Geometry check sheet. Reference: the model listing, model coordinates, mm. Face numbers are marked on the shaded views. A direction names the side the tool comes from. Give positions to 0.01 mm unless a question says otherwise; leave off trailing zeros. Write each loop counter-clockwise with the first axis right and the second up, starting at its lowest first coordinate (ties: lowest second). Pieces come first, ordered by that corner, then holes. Notation, with made-up numbers: (49, 4.25) -> (108, 4.25) arc R14 ccw to (108, 15.25) -> close; hole circle Ø5 at (-37, 86). An arc over 180 degrees is marked (long way). Use a Markdown table: item, result. Add a question column.
from build123d import *

# Parameters (mm, degrees)
SKETCH1_W                            = 40
SKETCH1_H                            = 10
BOSS_EXTRUDE1_DEPTH                  = 7.5
CBORE_FOR_M3_SHCS1_AT_2_COUNT        = 2
CBORE_FOR_M3_SHCS1_AT_2_PITCH        = 30
SKETCH4_W                            = 55
SKETCH4_H                            = 9.5
BOSS_EXTRUDE2_DEPTH                  = 40
BOSS_EXTRUDE3_DEPTH                  = 40
CUT_EXTRUDE1_DEPTH                   = 20.5
F_5_1_5_1_DIAMETER_HOLE1_D           = 5.1
F_5_1_5_1_DIAMETER_HOLE1_DEPTH       = 2.828427125
F_5_1_5_1_DIAMETER_HOLE1_CSINK_D     = 5.15
F_5_1_5_1_DIAMETER_HOLE1_CSINK_ANGLE = 90
CUT_EXTRUDE2_DEPTH                   = 20.5


with BuildPart() as part:
    # Sketch1 → Boss-Extrude1 (new body)
    with BuildSketch(Plane.XY):
        with Locations((20, -5)):
            Rectangle(SKETCH1_W, SKETCH1_H)
    extrude(amount=BOSS_EXTRUDE1_DEPTH)

    # Sketch3 → CBORE for M3 SHCS1 (revolve, cut)
    with BuildSketch(Plane(origin=(35, -5, 7.5), x_dir=(0, -1, 0), z_dir=(1, 0, 0))):
        Polygon((0, 0), (0, 7.5), (1.7, 7.5), (1.7, 3), (3.25, 3), (3.25, 0.025), (3.275, 0), align=None)
    cbore_for_m3_shcs1 = revolve(axis=Axis((35, -5, 13.85), (0, 0, -1)), mode=Mode.SUBTRACT)

    # CBORE for M3 SHCS1 at 2: CBORE for M3 SHCS1 ×2
    with Locations(*[(-i * CBORE_FOR_M3_SHCS1_AT_2_PITCH, 0, 0) for i in range(1, CBORE_FOR_M3_SHCS1_AT_2_COUNT)]):
        add(cbore_for_m3_shcs1, mode=Mode.SUBTRACT)

    # Sketch4 → Boss-Extrude2 (add)
    with BuildSketch(Plane.XY):
        with Locations((27.5, 4.75)):
            Rectangle(SKETCH4_W, SKETCH4_H)
    extrude(amount=BOSS_EXTRUDE2_DEPTH)

    # Sketch5 → Boss-Extrude3 (add)
    with BuildSketch(Plane(origin=(0, 9.5, 0), x_dir=(1, 0, 0), z_dir=(0, 1, 0))):
        Polygon((55, -10), (25, -40), (21, -40), (55, -6), align=None)
    extrude(amount=BOSS_EXTRUDE3_DEPTH)

    # Sketch7 → Cut-Extrude1 (cut, through all)
    with BuildSketch(Plane(origin=(0, 9.5, 0), x_dir=(1, 0, 0), z_dir=(0, 1, 0))):
        Polygon((55, -10), (25, -40), (55, -40), align=None)
    extrude(amount=-CUT_EXTRUDE1_DEPTH, mode=Mode.SUBTRACT)

    # Ø5.1 (5.1) Diameter Hole1
    with Locations(Plane(origin=(30.5, 0, 30.5), x_dir=(-0.707106781, 0, 0.707106781), z_dir=(-0.707106781, 0, -0.707106781))):
        with Locations((4.393398282, 29.5), (-25.606601718, 29.5)):
            CounterSinkHole(F_5_1_5_1_DIAMETER_HOLE1_D / 2, F_5_1_5_1_DIAMETER_HOLE1_CSINK_D / 2, depth=F_5_1_5_1_DIAMETER_HOLE1_DEPTH, counter_sink_angle=F_5_1_5_1_DIAMETER_HOLE1_CSINK_ANGLE)

    # Sketch11 → Cut-Extrude2 (cut, through all)
    with BuildSketch(Plane(origin=(0, 9.5, 0), x_dir=(1, 0, 0), z_dir=(0, 1, 0))):
        Polygon((0, -25), (0, -40), (15, -40), align=None)
    extrude(amount=-CUT_EXTRUDE2_DEPTH, mode=Mode.SUBTRACT)


solid = part.part
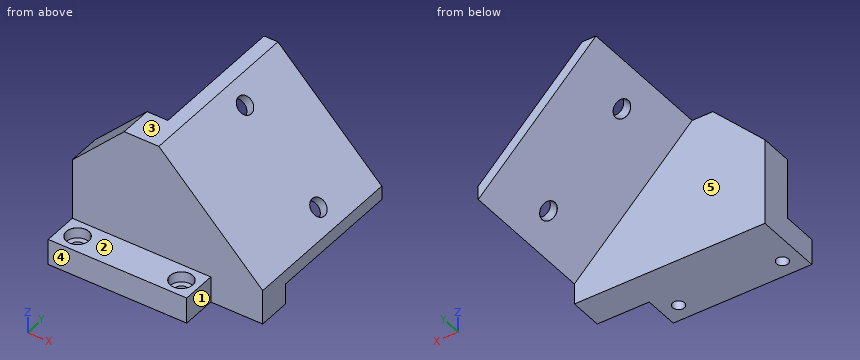
1) Tool access check on the marked faces 1, 2, 3, 4 and 5. Record the directions out of +Z, -Z, +X, -X, +Y, -Y that give a thin tool (end or side, any length) a straight path to the whole face; none if there is none.
2) Sectioned sample at D-D, the plane x = 35. Enter the section's corners in (y, z) (3 decimals).
3) Sectioned sample at B-B, the plane y = -5. Enter the section's corners in (x, z) (3 decimals), and give its area (3 significant figures).
4) Material ranges on probe 1 along X at (y, z) = (-5, 6); probe 2 along X at (y, z) = (-5, 2); probe 3 along Y at (x, z) = (35, 5), recorded low to high. Write a range as [from, to].
5) Gauge pin test, flat ends, axial feed: P1, Ø2, axis at x = 42.5, z = 21, coming from the -Y side; P2, Ø12, axis at x = 45, y = 9, coming from the +Z side; P3, Ø12, axis at x = 19, z = 17, coming from the +Y side. Record the tip position at first contact, or that the pin passes through.
6) Sectioned sample at C-C, the plane z = 9. Enter the section's corners in (x, y), and give its area (4 significant figures).
7) Sectioned sample at A-A, the plane x = 5. Enter the section's corners in (y, z) (3 decimals), and give its area (3 significant figures).
Check values:
| question | item | result |
|---|---|---|
| 1 | face 1 | +Z, -Z, +X, -Y |
| 1 | face 2 | +Z, +X, -X, -Y |
| 1 | face 3 | +Z, +X, -X, +Y, -Y |
| 1 | face 4 | +Z, -Z, +X, -X, -Y |
| 1 | face 5 | -Z, -X, +Y |
| 2 | outline | (-10, 0) -> (-6.7, 0) -> (-6.7, 4.5) -> (-8.25, 4.5) -> (-8.25, 7.475) -> (-8.275, 7.5) -> (-10, 7.5) -> close; (-3.3, 0) -> (9.5, 0) -> (9.5, 26) -> (49.5, 26) -> (49.5, 30) -> (0, 30) -> (0, 7.5) -> (-1.725, 7.5) -> (-1.75, 7.475) -> (-1.75, 4.5) -> (-3.3, 4.5) -> close |
| 3 | outline | (0, 0) -> (3.3, 0) -> (3.3, 4.5) -> (1.75, 4.5) -> (1.75, 7.475) -> (1.725, 7.5) -> (0, 7.5) -> close; (6.7, 0) -> (33.3, 0) -> (33.3, 4.5) -> (31.75, 4.5) -> (31.75, 7.475) -> (31.725, 7.5) -> (8.275, 7.5) -> (8.25, 7.475) -> (8.25, 4.5) -> (6.7, 4.5) -> close; (36.7, 0) -> (40, 0) -> (40, 7.5) -> (38.275, 7.5) -> (38.25, 7.475) -> (38.25, 4.5) -> (36.7, 4.5) -> close |
| 3 | area | 230 mm² |
| 4 | probe 1 | [0, 1.75], [8.25, 31.75], [38.25, 40] |
| 4 | probe 2 | [0, 3.3], [6.7, 33.3], [36.7, 40] |
| 4 | probe 3 | [-10, -8.25], [-1.75, 9.5] |
| 5 | P1 | y = 0 |
| 5 | P2 | z = 26 |
| 5 | P3 | y = 9.5 |
| 6 | outline | (0, 0) -> (55, 0) -> (55, 49.5) -> (52, 49.5) -> (52, 9.5) -> (0, 9.5) -> close |
| 6 | area | 642.5 mm² |
| 7 | outline | (-10, 0) -> (-6.7, 0) -> (-6.7, 4.5) -> (-8.25, 4.5) -> (-8.25, 7.475) -> (-8.275, 7.5) -> (-10, 7.5) -> close; (-3.3, 0) -> (9.5, 0) -> (9.5, 30) -> (0, 30) -> (0, 7.5) -> (-1.725, 7.5) -> (-1.75, 7.475) -> (-1.75, 4.5) -> (-3.3, 4.5) -> close |
| 7 | area | 325 mm² |
